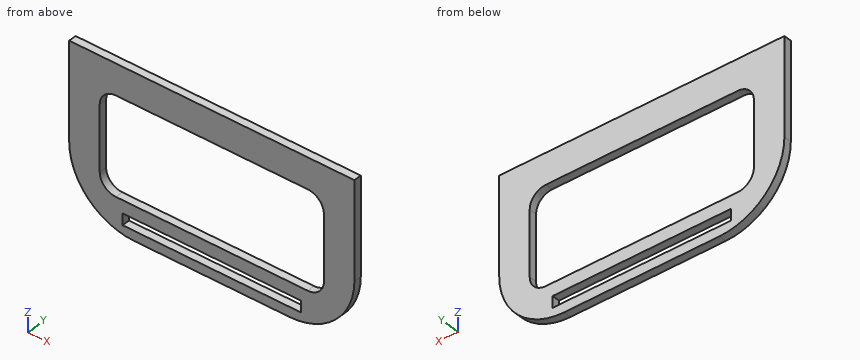
```python
from build123d import *

# Parameters (mm, degrees)
SKETCH1_W           = 8.795086316
SKETCH1_H           = 5
SKETCH1_W_2         = 5.5
SKETCH1_H_2         = 0.35
BOSS_EXTRUDE1_DEPTH = 0.24
FILLET1_R           = 2
SKETCH2_W           = 6.913332482
SKETCH2_H           = 3.007207861
CUT_EXTRUDE1_DEPTH  = 11.119839095
FILLET4_R           = 0.5


with BuildPart() as part:
    # Sketch1 → Boss-Extrude1 (new body)
    with BuildSketch(Plane(origin=(0, 0, 0), x_dir=(1, 0, 0), z_dir=(0, 1, 0))):
        with Locations((4.397543158, 2.5)):
            Rectangle(SKETCH1_W, SKETCH1_H)
        with Locations((4.397543158, 4.525)):
            Rectangle(SKETCH1_W_2, SKETCH1_H_2, mode=Mode.SUBTRACT)
    extrude(amount=BOSS_EXTRUDE1_DEPTH)

    # Fillet1
    fillet1_edges = [part.edges().sort_by_distance(p)[0] for p in [
        (0, 0.12, -5),
        (8.795086316, 0.12, -5),
    ]]
    fillet(fillet1_edges, radius=FILLET1_R)

    # Sketch2 → Cut-Extrude1 (cut, through all)
    with BuildSketch(Plane(origin=(0, 0.24, 0), x_dir=(1, 0, 0), z_dir=(0, 1, 0))):
        with Locations((4.397543158, 2.453300335)):
            Rectangle(SKETCH2_W, SKETCH2_H)
    extrude(amount=-CUT_EXTRUDE1_DEPTH, mode=Mode.SUBTRACT)

    # Fillet4
    fillet4_edges = [part.edges().sort_by_distance(p)[0] for p in [
        (0.940876917, 0.12, -0.949696404),
        (0.940876917, 0.12, -3.956904265),
        (7.854209399, 0.12, -3.956904265),
        (7.854209399, 0.12, -0.949696404),
    ]]
    fillet(fillet4_edges, radius=FILLET4_R)


solid = part.part
```
CAD build for the part. Positions are in the model's coordinates, mm. Round coordinates to 2 decimals unless told otherwise and drop trailing zeros. Order: outer loops, then holes, each group sorted by start corner. A loop starts at its lowest first (then second) coordinate and runs counter-clockwise, first axis right, second up. Notation, with made-up numbers: (-7.5, 34.5) -> (42.5, 34.5) arc R20 cw to (42.5, 63.5) -> close; hole circle Ø2 at (-32.75, -16.75). An arc over 180 degrees is marked (long way). Write item = value, one per line.
(1) Cut at A-A (y = 0.15). Write the cut outline in (x, z).
Answers follow:
outline = (0, -3) arc R2 ccw to (2, -5) -> (6.8, -5) arc R2 ccw to (8.8, -3) -> (8.8, 0) -> (0, 0) -> close; hole (0.94, -3.46) arc R0.5 ccw to (1.44, -3.96) -> (7.35, -3.96) arc R0.5 ccw to (7.85, -3.46) -> (7.85, -1.45) arc R0.5 ccw to (7.35, -0.95) -> (1.44, -0.95) arc R0.5 ccw to (0.94, -1.45) -> close; hole (1.65, -4.7) -> (7.15, -4.7) -> (7.15, -4.35) -> (1.65, -4.35) -> close
(2) Cut at B-B (x = 3.25). Write the cut outline in (y, z).
Answers follow:
outline = (0, -5) -> (0.24, -5) -> (0.24, -4.7) -> (0, -4.7) -> close; (0, -4.35) -> (0.24, -4.35) -> (0.24, -3.96) -> (0, -3.96) -> close; (0, -0.95) -> (0.24, -0.95) -> (0.24, 0) -> (0, 0) -> close
(3) Drill centre lines: L1, parallel to Z at x = 2, y = 0.2; L2, parallel to X at y = 0.05, z = -1.5; L3, parallel to X at y = 0.05, z = -3.45. Where is each one in solid material? Low to high.
Answers follow:
L1 = -5 to -4.7, -4.35 to -3.96, -0.95 to 0
L2 = 0 to 0.94, 7.85 to 8.8
L3 = 0.05 to 0.94, 7.85 to 8.74
(4) Cut at C-C (z = -3.6). Write the cut outline in (x, y).
Answers follow:
outline = (0.09, 0) -> (0.96, 0) -> (0.96, 0.24) -> (0.09, 0.24) -> close; (7.83, 0) -> (8.7, 0) -> (8.7, 0.24) -> (7.83, 0.24) -> close
(5) Cut at D-D (z = -1.2). Write the cut outline in (x, y).
Answers follow:
outline = (0, 0) -> (1.01, 0) -> (1.01, 0.24) -> (0, 0.24) -> close; (7.79, 0) -> (8.8, 0) -> (8.8, 0.24) -> (7.79, 0.24) -> close
